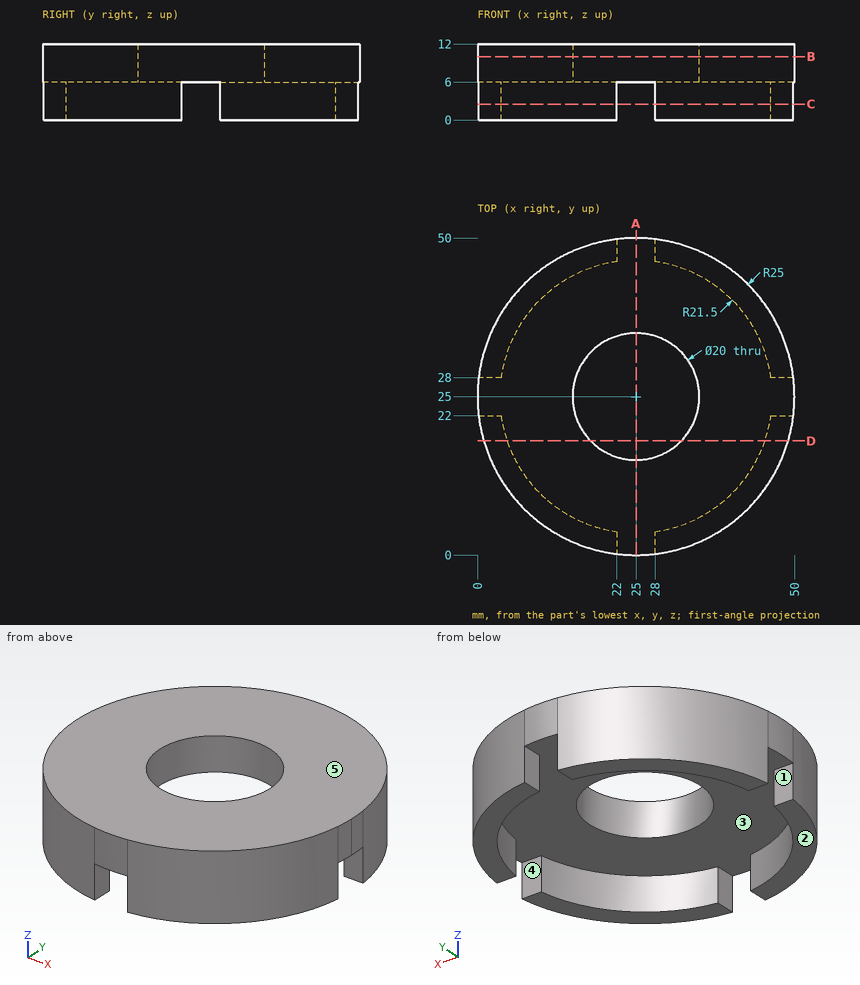
Input: dimensioned drawing with shaded views. Units: mm. Origin: part minimum x, y, z. A direction names the side the tool comes from. Coordinates: 2 decimals unless noted, no trailing zeros. Order: outer loops, then holes, each group sorted by start corner. A loop starts at its lowest first (then second) coordinate and runs counter-clockwise, first axis right, second up. Notation, with made-up numbers: (58.25, 87.25) - (105.25, 87.25) arc R24 cw to (105.25, 109.25) - close; hole circle Ø8 at (30, -6). An arc over 180 degrees is marked (long way). Put each result on its own line as item: value.
1. Cut plane D-D on y = 18. Return the cut outline in (x, z), then the cut area to 3 significant figures.
Report:
outline: (1, 0) - (4.67, 0) - (4.67, 6) - (17.86, 6) - (17.86, 12) - (1, 12) - close; (32.14, 6) - (45.33, 6) - (45.33, 0) - (49, 0) - (49, 12) - (32.14, 12) - close
area: 246 mm2
2. Contact query for flat-ended pins moving along their axis: pin 1 Ø4 at (y, z) = (49, 1.5) entering from +X; pin 2 Ø1.5 at (x, y) = (31.5, 21) entering from +Z; pin 3 Ø3 at (y, z) = (1.5, 3.5) entering from -X; pin 4 Ø1.1 at (x, z) = (47.5, 2) entering from -Y. Output: stop coordinate, or through.
Report:
pin 1: stops at x = 36.87
pin 2: passes through
pin 3: stops at x = 13.13
pin 4: stops at y = 13.03
3. Cut plane A-A on x = 25. Return the cut outline in (y, z).
Report:
outline: (0, 6) - (15, 6) - (15, 12) - (0, 12) - close; (35, 6) - (50, 6) - (50, 12) - (35, 12) - close
4. Cut plane C-C on z = 2.5. Return the cut outline in (x, y).
Report:
outline: (0.18, 22) arc R25 ccw to (22, 0.18) - (22, 3.71) arc R21.5 cw to (3.71, 22) - close; (0.18, 28) - (3.71, 28) arc R21.5 cw to (22, 46.29) - (22, 49.82) arc R25 ccw to start; (28, 0.18) arc R25 ccw to (49.82, 22) - (46.29, 22) arc R21.5 cw to (28, 3.71) - close; (28, 46.29) arc R21.5 cw to (46.29, 28) - (49.82, 28) arc R25 ccw to (28, 49.82) - close
5. Draft query along Y for the marked faces 1 and 2. Return one class per face: pulls with the +Y half, pulls with the -Y half, needs draft (parallel to the pull), parting line crosses it, or undercut.
Report:
face 1: undercut
face 2: needs draft
6. Reachability of the marked faces 3, 4 and 5 from +Z, -Z, +X, -X, +Y, -Y: full face, straight path, thin tool, end or side. Return the list, or none.
Report:
face 3: -Z
face 4: -Z, +X, -X
face 5: +Z, +X, -X, +Y, -Y
7. Cut plane B-B on z = 10. Return the cut outline in (x, y), then the cut area to 3 significant figures.
Report:
outline: circle Ø50 at (25, 25); hole circle Ø20 at (25, 25)
area: 1,650 mm2
8. Line query: line 1 along Z through (x, y) = (11.5, 15); line 2 along Y through (x, z) = (8, 2); line 3 along Y through (x, z) = (20, 4). Output: solid intervals per line, ascending.
Report:
line 1: z = 6 to 12
line 2: y = 6.67 to 11.84, 38.16 to 43.33
line 3: y = 0.51 to 4.09, 45.91 to 49.49
